Can you work these out from the model? Positions are in its coordinate system, mm. Face numbers are marked on the shaded views. A direction names the side the tool comes from. Give positions to 0.01 mm unless a question says otherwise; leave off trailing zeros. Loops run counter-clockwise (first coordinate to the right, second up) from the corner with the lowest first, then second, coordinate; pieces in that order, holes last. Notation, with made-up numbers: (10.5, -37) - (47.5, -37) arc R26 cw to (47.5, -6) - close; hole circle Ø11 at (-39.5, 33.5). An arc over 180 degrees is marked (long way). Write item = value, one per line.
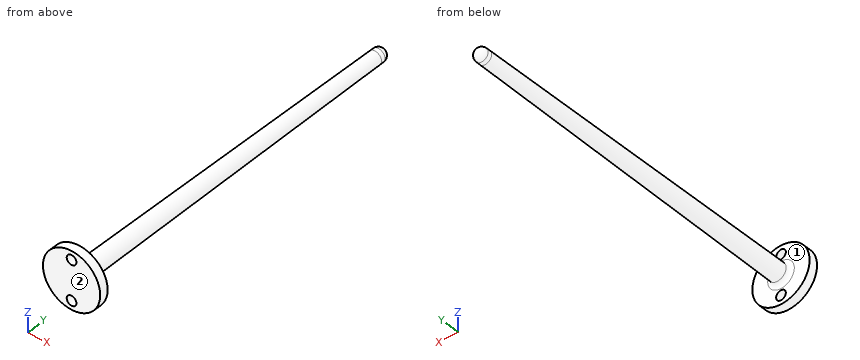
from build123d import *

# Parameters (mm, degrees)
SKETCH_1_R          = 6.5
EXTRUDE_1_DEPTH     = 2
SKETCH_2_R          = 1.1
CUT_EXTRUDE_1_DEPTH = 3


with BuildPart() as part:
    # 草图1 → 凸台-拉伸1 (new body)
    with BuildSketch(Plane(origin=(0, 0, 0), x_dir=(1, 0, 0), z_dir=(0, 1, 0))):
        Circle(SKETCH_1_R)
    extrude(amount=EXTRUDE_1_DEPTH)

    # 草图2 → 切除-拉伸1 (cut, through all)
    with BuildSketch(Plane(origin=(0, 2, 0), x_dir=(1, 0, 0), z_dir=(0, 1, 0))):
        with Locations((0, 4.5)):
            Circle(SKETCH_2_R)
        with Locations((0, -4.5)):
            Circle(SKETCH_2_R)
    extrude(amount=-CUT_EXTRUDE_1_DEPTH, mode=Mode.SUBTRACT)

    # 草图4 → 旋转1 (revolve)
    with BuildSketch(Plane.XY):
        with BuildLine():
            Line((1.50919925, 81.509373352), (2.02569692, 2.993421891))
            ThreePointArc((2.02569692, 2.993421891), (2.320898053, 2.290571318), (3.025675284, 2))
            Line((3.025675284, 2), (3, 2))
            Line((3, 2), (0, 2))
            Line((0, 2), (0, 83.938441204))
            ThreePointArc((0, 83.938441204), (1.05933326, 83.501690627), (1.503042796, 82.44525328))
            Line((1.503042796, 82.44525328), (1.50919925, 81.509373352))
        make_face()
    revolve(axis=Axis((0, 2, 0), (0, 1, 0)))


solid = part.part
Q1. Imagine slicing it at C-C, the plane y = 14.5. Write out the boundary of the cut face in (x, z).
Output:
outline = circle Ø3.9 at (0, 0)
Q2. Imagine slicing it at D-D, the plane y = 72. Write out the boundary of the cut face in (x, z).
Output:
outline = circle Ø3.14 at (0, 0)
Q3. Which directions (+Z, -Z, +X, -X, +Y, -Y) give clear straight access to the entire face, cutting with the end or side of a thin tool? Please do the marked faces 1 and 2.
Output:
face_1 = +Y
face_2 = +Z, -Z, +X, -X, -Y
Q4. For pin 1 (6 mm diameter, centred on x = 4.5, y = 40, fed in from -Z); pin 2 (2 mm diameter, centred on x = -4, z = -5, fed in from -Y); pin 3 (2.5 mm diameter, centred on x = 0, z = -4.5, fed in from +Y), each with a flat end and sliding along its axis, tell me the tip position at first contact or that it passes through.
Output:
pin_1 = -0.96
pin_2 = 0
pin_3 = 2
Q5. Imagine slicing it at B-B, the plane x = 0. Give the number of separate pieces and of enclosed holes in the cut face, then the cut area to 3 significant figures.
Output:
separate_pieces = 3
enclosed_holes = 0
area = 306 mm2
Q6. I need wall thicknesses on L1, parallel to Y at x = 5, z = 0.25; L2, parallel to X at y = 0.55, z = -4.5; L3, parallel to Y at x = 0.5, z = -0.75. Which ranges of each line are inside material? Lowest first, please.
Output:
L1 = 0 to 2
L2 = -4.69 to -1.1, 1.1 to 4.69
L3 = 0 to 83.64
Q7. Imagine slicing it at A-A, the plane z = -4.5. Write out the boundary of the cut face in (x, y), then the cut area to 3 significant figures.
Output:
outline = (-4.69, 0) - (-1.1, 0) - (-1.1, 2) - (-4.69, 2) - close; (1.1, 0) - (4.69, 0) - (4.69, 2) - (1.1, 2) - close
area = 14.4 mm2
